The listing builds one solid part. Answer for the finished solid, in the listing's coordinates (mm). Give positions to 0.01 mm unless a question says otherwise; leave off trailing zeros. Order: outer loops, then holes, each group sorted by start corner. A loop starts at its lowest first (then second) coordinate and runs counter-clockwise, first axis right, second up. Notation, with made-up numbers: (21, 44.25) - (79, 44.25) arc R27 cw to (79, 60.25) - close; hole circle Ø9 at (-37, 75.25). An arc over 180 degrees is marked (long way). Answer as a JSON object with one key per item and string values. Group by question number.
Q1. A cutting plane is placed at A-A, the plane y = 1.7. Give the vertices of the cut face in (x, z), and give its area (3 significant figures).
Q2. Given pin 1 (13 mm diameter, centred on x = 20, z = 20, fed in from -Y), flat-ended and moving along its own axis, determine where the tip first touches the part or whether it passes through.
Q3. A cutting plane is placed at B-B, the plane x = 65. Give the vertices of the cut face in (y, z), and give its area (3 significant figures).
Q4. Consider line 1 (X direction, y = 1.4, z = -20); line 2 (X direction, y = 1.25, z = -21); line 3 (Z direction, x = 22, y = 0.45). Determine where each line is inside the solid, lowest interval first.
Q5. A cutting plane is placed at D-D, the plane x = 21. Give the vertices of the cut face in (y, z), and give its area (3 significant figures).
Q6. A cutting plane is placed at C-C, the plane z = -10. Give the vertices of the cut face in (x, y).
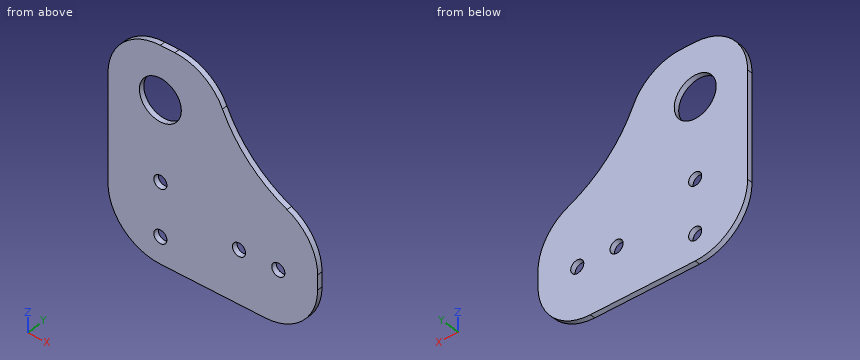
from build123d import *

# Parameters (mm, degrees)
SKETCH1_R           = 2.5
SKETCH1_W           = 40
SKETCH1_H           = 40
SKETCH1_R_2         = 8
BOSS_EXTRUDE1_DEPTH = 2
FILLET1_R           = 50
FILLET2_R           = 20


with BuildPart() as part:
    # Sketch1 → Boss-Extrude1 (new body)
    # profile 1 of 2: a face of its own
    with BuildSketch(Plane(origin=(0, 0, 0), x_dir=(1, 0, 0), z_dir=(0, 1, 0))):
        Polygon((80, 0), (80, 40), (0, 40), (0, 0), (40, 0), align=None)
        with Locations(Location((20, 10, 0), (0, 0, 270))):
            Circle(SKETCH1_R, mode=Mode.SUBTRACT)
        with Locations(Location((20, 30, 0), (0, 0, 270))):
            Circle(SKETCH1_R, mode=Mode.SUBTRACT)
        with Locations(Location((50, 20, 0), (0, 0, 270))):
            Circle(SKETCH1_R, mode=Mode.SUBTRACT)
        with Locations(Location((65, 20, 0), (0, 0, 270))):
            Circle(SKETCH1_R, mode=Mode.SUBTRACT)
    # profile 2 of 2: a face of its own
    with BuildSketch(Plane(origin=(0, 0, 0), x_dir=(1, 0, 0), z_dir=(0, 1, 0))):
        with Locations((20, -20)):
            Rectangle(SKETCH1_W, SKETCH1_H)
        with Locations(Location((20, -20, 0), (0, 0, 270))):
            Circle(SKETCH1_R_2, mode=Mode.SUBTRACT)
    extrude(amount=BOSS_EXTRUDE1_DEPTH)

    # Fillet1
    # the kernel refuses this fillet: 50 mm, written as the material it adds along each edge
    with BuildSketch(Plane(origin=(40, 0, 0), x_dir=(0, 0, 1), z_dir=(0, 1, 0))) as fillet1_piece_1:
        with BuildLine():
            CenterArc((49.154759474, 49.154759474), FILLET1_R, 190.550098012, 68.899803976)
            Line((0, 40), (0, 0))
            Line((0, 0), (40, 0))
        make_face()
    extrude(amount=2)

    # Fillet2
    fillet2_edges = [part.edges().sort_by_distance(p)[0] for p in [
        (80, 1, -40),
        (80, 1, 0),
        (40, 1, 40),
        (0, 1, 40),
        (0, 1, -40),
    ]]
    fillet(fillet2_edges, radius=FILLET2_R)


solid = part.part
Reply:
{
 "1": {"outline": "(0, -20) arc R20 ccw to (20, -40) - (60, -40) arc R20 ccw to (80, -20) - (80, -14.48) arc R20 ccw to (68.33, 3.7) arc R50 cw to (43.7, 28.33) arc R20 ccw to (25.52, 40) - (20, 40) arc R20 ccw to (0, 20) - close; hole circle Ø16 at (20, 20); hole circle Ø5 at (20, -30); hole circle Ø5 at (20, -10); hole circle Ø5 at (50, -20); hole circle Ø5 at (65, -20)", "area": "4,660 mm^2"},
 "2": {"pin 1": "passes through"},
 "3": {"outline": "(0, -39.36) - (2, -39.36) - (2, -22.5) - (0, -22.5) - close; (0, -17.5) - (2, -17.5) - (2, 5.38) - (0, 5.38) - close", "area": "79.5 mm^2"},
 "4": {"line 1": "x = 0 to 47.5, 52.5 to 62.5, 67.5 to 80", "line 2": "x = 0.03 to 47.71, 52.29 to 62.71, 67.29 to 79.97", "line 3": "z = -40 to -31.5, -28.5 to -11.5, -8.5 to 12.25, 27.75 to 40"},
 "5": {"outline": "(0, -40) - (2, -40) - (2, -32.29) - (0, -32.29) - close; (0, -27.71) - (2, -27.71) - (2, -12.29) - (0, -12.29) - close; (0, -7.71) - (2, -7.71) - (2, 12.06) - (0, 12.06) - close; (0, 27.94) - (2, 27.94) - (2, 40) - (0, 40) - close", "area": "110 mm^2"},
 "6": {"outline": "(0, 0) - (17.5, 0) - (17.5, 2) - (0, 2) - close; (22.5, 0) - (79.49, 0) - (79.49, 2) - (22.5, 2) - close"}
}
